Read the model definition and answer for the solid it produces. Units are mm, in the model's axes. Round coordinates to 2 decimals unless told otherwise and drop trailing zeros. Loops run counter-clockwise (first coordinate to the right, second up) from the corner with the lowest first, then second, coordinate; pieces in that order, holes last. Notation, with made-up numbers: M 62.25,58.5 L 67.25,58.5 A5 cw 67.25,63.5 Z; hole C -14,-20 d3. An arc over 180 degrees is marked long. Write each question's results on one line, items separated by ' | '.
```python
from build123d import *

# Parameters (mm, degrees)
SKETCH_1_R          = 1.6
EXTRUDE_1_DEPTH     = 2
CUT_EXTRUDE_1_DEPTH = 111.905365064
CHAMFER_1_SIZE      = 0.2
CHAMFER_1_SIZE2     = 0.1
CHAMFER_2_SIZE2     = 0.2
CHAMFER_2_SIZE      = 0.1


with BuildPart() as part:
    # Эскиз1 → Бобышка-Вытянуть1 (new body)
    with BuildSketch(Plane(origin=(0, 0, 0), x_dir=(1, 0, 0), z_dir=(0, 1, 0))):
        with BuildLine():
            Line((-75, 14), (-79.670248868, 1.785714286))
            ThreePointArc((-79.670248868, 1.785714286), (-80, 0), (-79.670248868, -1.785714286))
            Line((-79.670248868, -1.785714286), (-75, -14))
            Line((-75, -14), (25, -14))
            Line((25, -14), (29.670248868, -1.785714286))
            ThreePointArc((29.670248868, -1.785714286), (30, 0), (29.670248868, 1.785714286))
            Line((29.670248868, 1.785714286), (25, 14))
            Line((25, 14), (-75, 14))
        make_face()
        with Locations(Location((-75, 0, 0), (0, 0, 270))):
            Circle(SKETCH_1_R, mode=Mode.SUBTRACT)
        with Locations(Location((-25, 0, 0), (0, 0, 270))):
            Circle(SKETCH_1_R, mode=Mode.SUBTRACT)
        with Locations(Location((25, 0, 0), (0, 0, 270))):
            Circle(SKETCH_1_R, mode=Mode.SUBTRACT)
    extrude(amount=EXTRUDE_1_DEPTH)

    # Эскиз3 → Вырез-Вытянуть1 (cut, through all)
    with BuildSketch(Plane.ZY.offset(80)):
        Polygon((-13.8, 2), (-12.645299462, 0), (-14, 0), (-14, 2), align=None)
        Polygon((13.8, 2), (12.645299462, 0), (14, 0), (14, 2), align=None)
    extrude(amount=-CUT_EXTRUDE_1_DEPTH, mode=Mode.SUBTRACT)

    # Фаска1
    chamfer_1_edges = [part.edges().sort_by_distance(p)[0] for p in [
        (-25, 2, -13.8),
    ]]
    chamfer_1_side = [part.faces().sort_by_distance(p)[0] for p in [
        (-25, 0.998536994, -13.221805064),
    ]]
    chamfer(chamfer_1_edges, length=CHAMFER_1_SIZE, length2=CHAMFER_1_SIZE2, reference=chamfer_1_side[0])

    # Фаска2
    chamfer_2_edges = [part.edges().sort_by_distance(p)[0] for p in [
        (-25, 2, 13.8),
    ]]
    chamfer_2_side = [part.faces().sort_by_distance(p)[0] for p in [
        (-25, 2, 13.798),
    ]]
    chamfer(chamfer_2_edges, length=CHAMFER_2_SIZE - 0.0001, length2=CHAMFER_2_SIZE2 - 0.0001, reference=chamfer_2_side[0])  # a hair under: the kernel refuses the full size


solid = part.part
```
1. Determine the mould class of faces 1 (the face through (-26, 2, -3)), 2 (the face through (-23.414, 0.986, -0.208)), 3 (the face through (-77.36, 0.99, -7.83)), 4 (the face through (-73.414, 0.986, -0.208)) for opening direction Z: released by +Z, released by -Z, zero draft, split by the parting line, or undercut.
Completed:
face 1: zero draft | face 2: undercut | face 3: released by -Z | face 4: undercut
2. Find section C-C, the plane y = 1.25. Give the vertices of the cut face in (x, z), then the cut area to 3 significant figures.
Completed:
outline: M -79.67,-1.79 L -75.24,-13.37 L 25.24,-13.37 L 29.67,-1.79 A5 ccw 29.67,1.79 L 25.24,13.37 L -75.24,13.37 L -79.67,1.79 A5 ccw Z; hole C -75,0 d3.2; hole C -25,0 d3.2; hole C 25,0 d3.2 | area: 2,800 mm2
3. Find section A-A, the plane x = -25. Give the vertices of the cut face in (y, z).
Completed:
outline: M 0,-12.65 L 1.83,-13.7 L 2,-13.7 L 2,-1.6 L 0,-1.6 Z; M 0,1.6 L 2,1.6 L 2,13.7 L 1.83,13.7 L 0,12.65 Z
4. Given P1, Ø3, axis at x = -25, z = 0, coming from the +Y side, flat-ended and moving along its own axis, determine where the tip first touches the part or whether it passes through.
Completed:
P1: passes through
5. Find the intervals of material crossed by L1, parallel to X at y = 0.7, z = 0; L2, parallel to X at y = 1, z = 0.75; L3, parallel to Z at x = -75, y = 1.45, in increasing order.
Completed:
L1: x = -80 to -76.6, -73.4 to -26.6, -23.4 to 23.4, 26.6 to 30 | L2: x = -79.94 to -76.41, -73.59 to -26.41, -23.59 to 23.59, 26.41 to 29.94 | L3: z = -13.48 to -1.6, 1.6 to 13.48
6. Find section B-B, the plane z = 0. Give the vertices of the cut face in (x, y).
Completed:
outline: M -80,0 L -76.6,0 L -76.6,2 L -80,2 Z; M -73.4,0 L -26.6,0 L -26.6,2 L -73.4,2 Z; M -23.4,0 L 23.4,0 L 23.4,2 L -23.4,2 Z; M 26.6,0 L 30,0 L 30,2 L 26.6,2 Z
7. Find section D-D, the plane x = -51.5. Give the vertices of the cut face in (y, z), then the cut area to 3 significant figures.
Completed:
outline: M 0,-12.65 L 1.83,-13.7 L 2,-13.7 L 2,13.7 L 1.83,13.7 L 0,12.65 Z | area: 52.9 mm2
